Read the model definition and answer for the solid it produces. Units are mm, in the model's axes. Face numbers are marked on the shaded views. A direction names the side the tool comes from. Give positions to 0.01 mm unless a question says otherwise; leave off trailing zeros. Loops run counter-clockwise (first coordinate to the right, second up) from the corner with the lowest first, then second, coordinate; pieces in that order, holes last. Notation, with made-up numbers: (86, 9.5) -> (92, 9.5) arc R21 cw to (92, 23.5) -> close; hole circle Ø11 at (15, 89). An arc over 180 degrees is marked (long way). One line per item, written item: value. Start each with the question number.
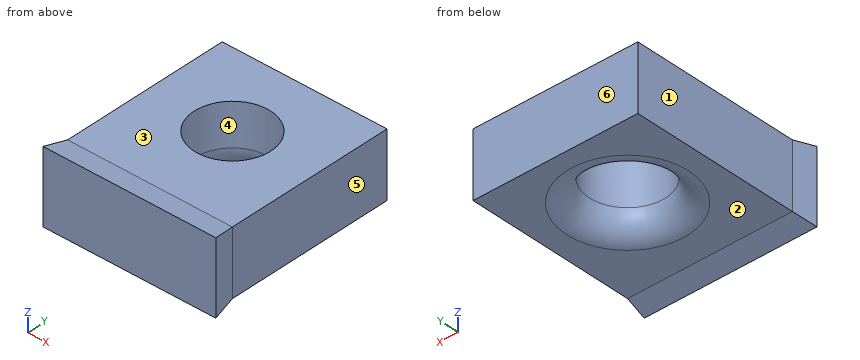
Autodesk Inventor part; units mm, degrees
ref_plane "YZ Plane" through (0, 0, 0) normal (1, 0, 0) x (0, 1, 0)
ref_plane "XZ Plane" through (0, 0, 0) normal (0, 1, 0) x (-1, 0, 0)
ref_plane "XY Plane" through (0, 0, 0) normal (0, 0, 1) x (1, 0, 0)
sketch "Sketch1" plane through (0, 0, 0) normal (0, 1, 0) x (-1, 0, 0)
  point P0 (0, 0)
sketch "Sketch2" plane through (0, 0, 0) normal (0, 1, 0) x (-1, 0, 0)
  line L0 (0, 0) -> (14.6, 0)
  line L1 (14.6, 0) -> (14.6, -5.75)
  line L2 (14.6, -5.75) -> (0, -5.75)
  line L3 (0, -5.75) -> (0, 0)
  dimension "d0" = 14.6
  dimension "d1" = 5.75
extrude "Extrusion1" add sketch "Sketch2" along normal blind 15 and the other way blind 2 draft 10
sketch "Sketch3" plane through (-14.6, 0, 0) normal (0, 0, 1) x (1, 0, 0)
  line L0 (0, 15) -> (14.6, 15)
  point P0 (14.6, 0)
  point P1 (7.3, 8)
  point P2 (7.3, 15)
  dimension "d6" = 7
hole "Hole1" at (-7.3, 8, 0) direction (0, 0, -1) diameter 6.7564 depth 12.7 tip angle 118
fillet "Fillet1" radius 2 1 edges at (-7.3, 11.3782, -5.75)
properties part number "Support Hole"
Item 1: Section B-B, the plane x = -7.3 is taken. Determine the outline of the cut face in (y, z).
Item 2: For the marked faces 1, 2 and 3, determine the directions among +Z, -Z, +X, -X, +Y, -Y from which every point of the face is accessible in a straight line to the end or side of a thin tool.
Item 3: Section A-A, the plane y = 8 is taken. Determine the outline of the cut face in (x, z).
Item 4: Determine the mould class of the marked faces 4, 5 and 6 for opening direction X: pulls with the +X half, pulls with the -X half, needs draft (parallel to the pull), parting line crosses it, or undercut.
Item 5: Consider L1, parallel to Y at x = -7.3, z = -1.6; L2, parallel to X at y = 8, z = -2.7; L3, parallel to Z at x = -13.25, y = 0.75. Determine where each line is inside the solid, lowest interval first. Write a range as [from, to].
Item 6: Section C-C, the plane z = -1.75 is taken. Determine the outline of the cut face in (x, y).
Item 7: Flat-ended cylindrical pins translate along their axes: pin 1 (9 mm diameter, centred on x = -7.3, y = 8, fed in from +Z); pin 2 (1.5 mm diameter, centred on x = -11.5, y = 9, fed in from -Z); pin 3 (1.5 mm diameter, centred on y = 13, z = -4, fed in from +X). Find the tip coordinate at first contact, or state that the pin passes through.
Item 8: Section D-D, the plane x = -13.5 is taken. Determine the outline of the cut face in (y, z), plus the area to 3 significant figures.
Computed values:
1. outline: (-2, -6.1) -> (0, -5.75) -> (2.62, -5.75) arc R2 ccw to (4.62, -3.75) -> (4.62, 0) -> (0, 0) -> (-2, 0.35) -> close; (11.38, -3.75) arc R2 ccw to (13.38, -5.75) -> (15, -5.75) -> (15, 0) -> (11.38, 0) -> close
2. face 1: +Z, -Z, -X, +Y
2. face 2: -Z, +X, -X, +Y
2. face 3: +Z, +X, -X, +Y
3. outline: (-14.6, -5.75) -> (-12.68, -5.75) arc R2 ccw to (-10.68, -3.75) -> (-10.68, 0) -> (-14.6, 0) -> close; (-3.92, -3.75) arc R2 ccw to (-1.92, -5.75) -> (0, -5.75) -> (0, 0) -> (-3.92, 0) -> close
4. face 4: undercut
4. face 5: pulls with the +X half
4. face 6: needs draft
5. L1: [-2, 4.62], [11.38, 15]
5. L2: [-14.6, -10.68], [-3.92, 0]
5. L3: [-5.75, 0]
6. outline: (-14.95, -2) -> (0.35, -2) -> (0, 0) -> (0, 15) -> (-14.6, 15) -> (-14.6, 0) -> close; hole circle Ø6.76 at (-7.3, 8)
7. pin 1: z = 0
7. pin 2: z = -5.73
7. pin 3: x = 0
8. outline: (-2, -6.1) -> (0, -5.75) -> (15, -5.75) -> (15, 0) -> (0, 0) -> (-2, 0.35) -> close
8. area: 98.5 mm²
